The listing builds one solid part. Answer for the finished solid, in the listing's coordinates (mm). Face numbers are marked on the shaded views. A direction names the side the tool comes from. Round coordinates to 2 decimals unless told otherwise and drop trailing zeros. Write each loop counter-clockwise with the first axis right and the second up, starting at its lowest first coordinate (ties: lowest second). Pieces come first, ordered by that corner, then holes. Notation, with made-up numbers: (48.25, -10.5) - (69.25, -10.5) arc R20 ccw to (69.25, -2.5) - close; hole circle Ø7 at (72.25, -28). An arc over 180 degrees is marked (long way). Return JSON: item names as keys, results as strings. Group by question number.
Autodesk Inventor part; units mm, degrees
ref_plane "YZ Plane" through (0, 0, 0) normal (1, 0, 0) x (0, 1, 0)
ref_plane "XZ Plane" through (0, 0, 0) normal (0, 1, 0) x (-1, 0, 0)
ref_plane "XY Plane" through (0, 0, 0) normal (0, 0, 1) x (1, 0, 0)
sketch "mounting sheet" plane through (0, 0, 0) normal (0, 1, 0) x (-1, 0, 0)
  line L0 (9.4, -11.43) -> (-9.4, -11.43)
  line L1 (-9.4, -11.43) -> (-9.4, 11.43)
  line L2 (-9.4, 11.43) -> (9.4, 11.43)
  line L3 (9.4, 11.43) -> (9.4, -11.43)
  line L4 (9.4, -11.43) -> (-9.4, 11.43) construction
  line L5 (-9.4, -11.43) -> (9.4, 11.43) construction
  point P0 (0, 0)
  dimension "d0" = 18.8
  dimension "d1" = 22.86
extrude "mounting" add sketch "mounting sheet" along normal blind 1.02
sketch "Sketch2" plane through (0, 1.02, 0) normal (0, 1, 0) x (1, 0, 0)
  line L0 (-9.4, 11.43) -> (-9.4, -11.43) construction
  line L1 (-9.4, -8.33) -> (9.4, -8.33) construction
  line L2 (9.4, -11.43) -> (9.4, 11.43) construction
  line L3 (-9.4, -11.43) -> (9.4, -11.43) construction
  point P0 (0, 0)
  point P1 (-6.3, -8.33)
  point P2 (6.3, -8.33)
  dimension "d10" = 3.1
  dimension "d11" = 3.1
  dimension "d12" = 12.6
hole "Hole1" at (-6.3, 1.02, 8.33) at (6.3, 1.02, 8.33) direction (0, -1, 0) diameter 2.69 end through all
sketch "Sketch4" plane through (0, 1.02, 0) normal (0, 1, 0) x (1, 0, 0)
  line L0 (9.4, 11.43) -> (-9.4, 11.43)
  line L1 (9.4, -11.43) -> (9.4, 11.43)
  line L2 (-9.4, 11.43) -> (9.4, 11.43)
  line L3 (9.4, 11.43) -> (9.4, -5.23)
  line L4 (9.4, -5.23) -> (-9.4, -5.23)
  line L5 (-9.4, -5.23) -> (-9.4, 11.43)
  line L6 (-9.4, -11.43) -> (9.4, -11.43)
  point P0 (0, 0)
  dimension "d21" = 6.2
extrude "Extrusion2" add sketch "Sketch4" along normal blind 12.7
sketch "Sketch5" plane through (-9.4, 1.02, 5.23) normal (0, 0, 1) x (1, 0, 0)
  line L0 (18.8, 12.7) -> (0, 12.7) construction
  line L1 (9.4, 12.7) -> (9.4, 0) construction
  line L2 (0, 0) -> (18.8, 0) construction
  line L3 (18.8, -1.02) -> (18.8, 12.7) construction
  line L4 (0, -1.02) -> (0, 12.7) construction
  line L5 (18.8, 6.35) -> (0, 6.35) construction
  point P0 (9.4, -1.02)
  point P1 (9.4, 6.35)
  dimension "d25" = 7.37
hole "Hole2" at (0, 7.37, 5.23) direction (0, 0, -1) diameter 3 depth 5 tip angle 118
sketch "Sketch6" plane through (9.4, 0, 11.43) normal (1, 0, 0) x (0, 0, -1)
  line L0 (6.2, 1.02) -> (6.2, 13.72) construction
  line L1 (6.2, 7.37) -> (22.8459, 7.37) construction
  line L2 (6.2, 13.72) -> (22.86, 13.72) construction
  line L3 (0, 0) -> (22.86, 0) construction
  line L4 (10.26, 13.72) -> (10.26, 0) construction
  point P0 (11.43, 0)
  point P1 (10.26, 7.37)
  dimension "d33" = 4.06
  dimension "d34" = 7.37
hole "Hole3" at (9.4, 7.37, 1.17) direction (-1, 0, 0) diameter 3 end through all
sketch "Sketch7" plane through (0, 13.72, 0) normal (0, 1, 0) x (1, 0, 0)
  line L0 (-9.4, 11.43) -> (9.4, 11.43) construction
  line L1 (9.4, 11.43) -> (9.4, -5.23) construction
  line L2 (9.4, -5.23) -> (-9.4, -5.23) construction
  line L3 (-9.4, -5.23) -> (-9.4, 11.43) construction
  line L4 (-9.4, 11.43) -> (-9.4, -5.23)
  line L5 (9.4, -5.23) -> (9.4, 11.43)
  line L6 (9.4, 11.43) -> (-9.4, 11.43)
  line L7 (-9.4, -5.23) -> (9.4, -5.23)
  point P0 (0, 0)
  point P1 (0, -5.23)
properties part number "ZX10-2-12-S+"
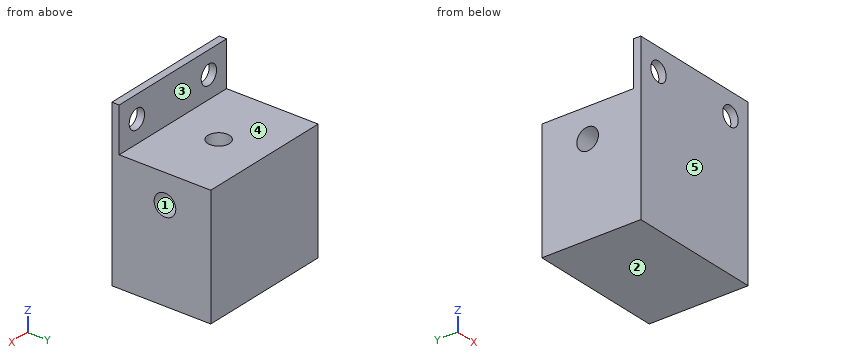
(1) Find section B-B (z = 8.33). Write down the section's boundary in (x, y) (3 decimals), plus the area to 3 significant figures.
(2) For the marked faces 4 and 5, determine the directions among +Z, -Z, +X, -X, +Y, -Y from which every point of the face is accessible in a straight line to the end or side of a thin tool.
(3) Consider line 1 (X direction, y = 0.45, z = 8.33) (3 decimals); line 2 (Z direction, x = 6.3, y = 0.75) (3 decimals); line 3 (Z direction, x = -4.5, y = 7.37). Determine where each line is inside the solid, lowest interval first.
(4) Determine the mould class of the marked faces 1, 2 and 3 for opening direction Z: +Z half, -Z half, draft (parallel to the pull), parting line (faces both ways), or undercut.
(5) Find section A-A (x = -6.3). Write down the section's boundary in (y, z) (3 decimals).
(6) Find section D-D (y = 9.75). Write down the section's boundary in (x, z).
(7) Find section C-C (x = -3). Write down the section's boundary in (y, z), plus the area to 3 significant figures.
(8) Flat-ended cylindrical pins translate along their axes: pin 1 (2 mm diameter, centred on x = 3.5, y = 4.5, fed in from +Z); pin 2 (3 mm diameter, centred on x = 4, z = 9.5, fed in from +Y); pin 3 (2.5 mm diameter, centred on x = 0, y = 7.37, fed in from +Z). Find the tip coordinate at first contact, or state that the pin passes through.
Check sheet entries:
{
 "1": {"outline": "(-9.4, 0) - (-7.645, 0) - (-7.645, 1.02) - (-9.4, 1.02) - close; (-4.955, 0) - (4.955, 0) - (4.955, 1.02) - (-4.955, 1.02) - close; (7.645, 0) - (9.4, 0) - (9.4, 1.02) - (7.645, 1.02) - close", "area": "13.7 mm^2"},
 "2": {"face 4": "+Z, +X, -X, +Y", "face 5": "+Z, -Z, +X, -X, -Y"},
 "3": {"line 1": "x = -9.4 to -7.645, -4.955 to 4.955, 7.645 to 9.4", "line 2": "z = -11.43 to 6.985, 9.675 to 11.43", "line 3": "z = -11.43 to -0.33, 2.67 to 5.23"},
 "4": {"face 1": "undercut", "face 2": "-Z half", "face 3": "draft"},
 "5": {"outline": "(0, -11.43) - (13.72, -11.43) - (13.72, 5.23) - (1.02, 5.23) - (1.02, 6.985) - (0, 6.985) - close; (0, 9.675) - (1.02, 9.675) - (1.02, 11.43) - (0, 11.43) - close; hole circle Ø3 at (7.37, 1.17)"},
 "6": {"outline": "(-9.4, -11.43) - (9.4, -11.43) - (9.4, 5.23) - (-9.4, 5.23) - close"},
 "7": {"outline": "(0, -11.43) - (13.72, -11.43) - (13.72, 5.23) - (1.02, 5.23) - (1.02, 11.43) - (0, 11.43) - close; hole circle Ø3 at (7.37, 1.17)", "area": "228 mm^2"},
 "8": {"pin 1": "stops at z = 5.23", "pin 2": "stops at y = 1.02", "pin 3": "stops at z = 0.08"}
}
